```python
from build123d import *
from build123d.topology import SkipClean

# Parameters (mm, degrees)
SKETCH1_R               = 3.429
SKETCH1_R_2             = 2.286
BOSS_EXTRUDE1_DEPTH     = 3.556
BOSS_EXTRUDE2_START     = -1.27
BOSS_EXTRUDE2_DEPTH     = 1.27
BOSS_EXTRUDE3_START     = -1.27
SKETCH2_3_R             = 2.286
SKETCH2_3_R_2           = 1.27
BOSS_EXTRUDE3_DEPTH     = 0.254
SKETCH3_R               = 0.508
CUT_EXTRUDE1_DEPTH      = 17.020635974
LPATTERN1_COUNT         = 6
LPATTERN1_PITCH         = 1.778
CUT_EXTRUDE2_DEPTH      = 17.020635974
CUT_EXTRUDE2_DEPTH_BACK = 17.020635974
SKETCH4_W               = 4.326879353
SKETCH4_H               = 6.724216597
BOSS_EXTRUDE4_START     = 2.286
SKETCH5_R               = 0.508
BOSS_EXTRUDE4_DEPTH     = 1.27
COMBINE1_OUTLINE_R      = 0.508
COMBINE1_OUTLINE_R_2    = 1.27
COMBINE1_DEPTH          = 3.556
SKETCH6_W               = 6.35
SKETCH6_H               = 12.7
BOSS_EXTRUDE5_DEPTH     = 1.27
BOSS_EXTRUDE6_START     = -1.27
SKETCH6_2_W             = 6.35
SKETCH6_2_H             = 12.7
BOSS_EXTRUDE6_DEPTH     = 1.27
FILLET1_R               = 1.27


# Read off the part's stored shape, not the designer's step: Combine1
with BuildPart() as part:
    # Sketch1 → Boss-Extrude1 (new body)
    with BuildSketch(Plane(origin=(0, 0, 0), x_dir=(1, 0, 0), z_dir=(0, 1, 0))):
        with Locations(Location((0, 0, 0), (0, 0, 270))):
            Circle(SKETCH1_R)
        with Locations(Location((0, 0, 0), (0, 0, 270))):
            Circle(SKETCH1_R_2, mode=Mode.SUBTRACT)
    extrude(amount=BOSS_EXTRUDE1_DEPTH)

    # Sketch2 → Boss-Extrude2 (add)
    with BuildSketch(Plane(origin=(0, 3.556, 0), x_dir=(1, 0, 0), z_dir=(0, 1, 0)).offset(BOSS_EXTRUDE2_START)):
        with BuildLine():
            ThreePointArc((-2.54, 2.303571358), (-1.389081498, 3.135042837), (0, 3.429))
            Line((0, 3.429), (0, 15.24))
            ThreePointArc((0, 15.24), (-0.835660201, 14.92028345), (-1.244511661, 14.124427226))
            Line((-1.244511661, 14.124427226), (-2.54, 2.303571358))
        make_face()
        with BuildLine():
            Line((0, 15.24), (0, 3.429))
            ThreePointArc((0, 3.429), (1.389081498, 3.135042837), (2.54, 2.303571358))
            Line((2.54, 2.303571358), (1.244511661, 14.124427226))
            ThreePointArc((1.244511661, 14.124427226), (0.835660201, 14.92028345), (0, 15.24))
        make_face()
    extrude(amount=BOSS_EXTRUDE2_DEPTH)

    # Sketch2<3> → Boss-Extrude3 (add)
    with BuildSketch(Plane(origin=(0, 3.556, 0), x_dir=(1, 0, 0), z_dir=(0, 1, 0)).offset(BOSS_EXTRUDE3_START)):
        with Locations(Location((0, 0, 0), (0, 0, 270))):
            Circle(SKETCH2_3_R)
        with Locations(Location((0, 0, 0), (0, 0, 270))):
            Circle(SKETCH2_3_R_2, mode=Mode.SUBTRACT)
    extrude(amount=BOSS_EXTRUDE3_DEPTH)

    # Sketch3 → Cut-Extrude1 (cut, through all)
    with BuildSketch(Plane(origin=(0, 3.556, 0), x_dir=(1, 0, 0), z_dir=(0, 1, 0))):
        with Locations(Location((0, 5.08, 0), (0, 0, 270))):
            Circle(SKETCH3_R)
    cut_extrude1 = extrude(amount=-CUT_EXTRUDE1_DEPTH, mode=Mode.SUBTRACT)

    # LPattern1: Cut-Extrude1 ×6
    with Locations(*[(0, 0, -i * LPATTERN1_PITCH) for i in range(1, LPATTERN1_COUNT)]):
        add(cut_extrude1, mode=Mode.SUBTRACT)

    # Sketch4 → Cut-Extrude2 (cut, two sides: drawn at the far end of the back side and taken through both)
    with BuildSketch(Plane(origin=(0, 0, 0), x_dir=(0, 0, -1), z_dir=(1, 0, 0)).offset(-CUT_EXTRUDE2_DEPTH_BACK)):
        with Locations((-2.163439677, 3.362108299)):
            Rectangle(SKETCH4_W, SKETCH4_H)
    extrude(amount=CUT_EXTRUDE2_DEPTH + CUT_EXTRUDE2_DEPTH_BACK, mode=Mode.SUBTRACT)

    # Mirror1: part across plane


with BuildPart() as part_1:
    with SkipClean():  # the faces are left unmerged after this step: merging them gives an invalid solid
        add(part.part)
        add(part.part.mirror(Plane.XY))


with BuildPart() as body_2:
    # Sketch5 → Boss-Extrude4 (new body)
    with BuildSketch(Plane(origin=(0, 0, 0), x_dir=(1, 0, 0), z_dir=(0, 1, 0)).offset(BOSS_EXTRUDE4_START)):
        Polygon((3.175, 16.51), (15.875, 12.7), (3.175, 8.89), (3.175, 3.81), (-3.175, 3.81), (-3.175, 16.51), align=None)
        with Locations(Location((4.191, 12.7, 0), (0, 0, 270))):
            Circle(SKETCH5_R, mode=Mode.SUBTRACT)
        with Locations(Location((5.969, 12.7, 0), (0, 0, 270))):
            Circle(SKETCH5_R, mode=Mode.SUBTRACT)
        with Locations(Location((7.747, 12.7, 0), (0, 0, 270))):
            Circle(SKETCH5_R, mode=Mode.SUBTRACT)
        with Locations(Location((9.525, 12.7, 0), (0, 0, 270))):
            Circle(SKETCH5_R, mode=Mode.SUBTRACT)
        with Locations(Location((11.303, 12.7, 0), (0, 0, 270))):
            Circle(SKETCH5_R, mode=Mode.SUBTRACT)
    extrude(amount=BOSS_EXTRUDE4_DEPTH)


with BuildPart() as combine1_tool:
    # Combine1 outline → Combine1 (new body)
    with BuildSketch(Plane(origin=(0, 0, 0), x_dir=(1, 0, 0), z_dir=(0, 1, 0))):
        with BuildLine():
            ThreePointArc((2.54, -2.303571358), (3.429, 0), (2.54, 2.303571358))
            Line((2.54, 2.303571358), (1.244511661, 14.124427226))
            ThreePointArc((1.244511661, 14.124427226), (0, 15.24), (-1.244511661, 14.124427226))
            Line((-1.244511661, 14.124427226), (-2.54, 2.303571358))
            ThreePointArc((-2.54, 2.303571358), (-3.429, 0), (-2.54, -2.303571358))
            Line((-2.54, -2.303571358), (-1.244511661, -14.124427226))
            ThreePointArc((-1.244511661, -14.124427226), (0, -15.24), (1.244511661, -14.124427226))
            Line((1.244511661, -14.124427226), (2.54, -2.303571358))
        make_face()
        with Locations((0, -5.08)):
            Circle(COMBINE1_OUTLINE_R, mode=Mode.SUBTRACT)
        with Locations((0, -13.97)):
            Circle(COMBINE1_OUTLINE_R, mode=Mode.SUBTRACT)
        with Locations((0, -12.192)):
            Circle(COMBINE1_OUTLINE_R, mode=Mode.SUBTRACT)
        with Locations((0, -10.414)):
            Circle(COMBINE1_OUTLINE_R, mode=Mode.SUBTRACT)
        with Locations((0, -8.636)):
            Circle(COMBINE1_OUTLINE_R, mode=Mode.SUBTRACT)
        with Locations((0, -6.858)):
            Circle(COMBINE1_OUTLINE_R, mode=Mode.SUBTRACT)
        Circle(COMBINE1_OUTLINE_R_2, mode=Mode.SUBTRACT)
    extrude(amount=COMBINE1_DEPTH)


with BuildPart() as part_2:
    add(part_1.part)

    # Combine1: cut by combine1_tool
    add(combine1_tool.part, mode=Mode.SUBTRACT)


with BuildPart() as body_2_1:
    add(body_2.part)

    # Combine1: cut by combine1_tool
    add(combine1_tool.part, mode=Mode.SUBTRACT)

    # Sketch6 → Boss-Extrude5 (add)
    with BuildSketch(Plane.XZ.offset(-2.286)):
        with Locations((0, -10.16)):
            Rectangle(SKETCH6_W, SKETCH6_H)
    extrude(amount=BOSS_EXTRUDE5_DEPTH)

    # Sketch6<2> → Boss-Extrude6 (add)
    with BuildSketch(Plane.XZ.offset(-2.286).offset(BOSS_EXTRUDE6_START)):
        with Locations((0, -10.16)):
            Rectangle(SKETCH6_2_W, SKETCH6_2_H)
    extrude(amount=-BOSS_EXTRUDE6_DEPTH)

    # Fillet1
    fillet1_edges = [body_2_1.edges().sort_by_distance(p)[0] for p in [
        (15.875, 2.921, -12.7),
    ]]
    fillet(fillet1_edges, radius=FILLET1_R)


solid = body_2_1.part
```
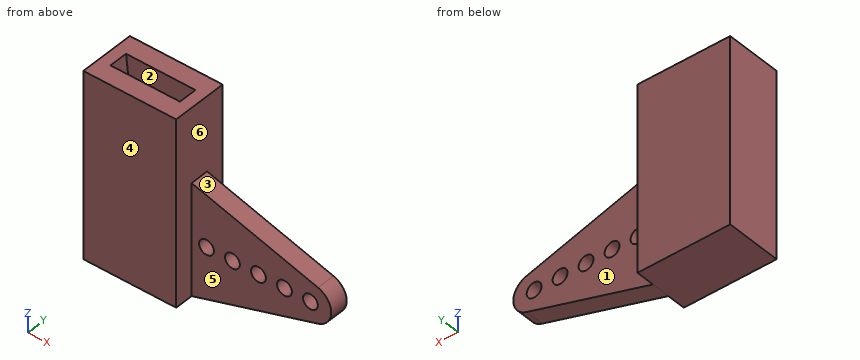
Geometry check sheet. Reference: the model listing, model coordinates, mm. Face numbers are marked on the shaded views. A direction names the side the tool comes from. Coordinates: 2 decimals unless noted, no trailing zeros. Loops run counter-clockwise (first coordinate to the right, second up) from the corner with the lowest first, then second, coordinate; pieces in that order, holes last.
Item 1: Sectioned sample at B-B, the plane y = 3. Record the boundary of the cut face in (x, z) (3 decimals), then the cut area to 3 significant figures.
Item 2: Sectioned sample at C-C, the plane x = 11. Record the boundary of the cut face in (y, z).
Item 3: Go/stop test with flat-tipped pins: pin 1 Ø6 at (x, z) = (9.5, -11.5) entering from +Y; pin 2 Ø1 at (x, y) = (5.5, 3) entering from -Z; pin 3 Ø1.3 at (x, z) = (11.303, -12.7) entering from -Y. Record where each tip stops, or that it passes through.
Item 4: Access from +Z, -Z, +X, -X, +Y, -Y to the whole of each face (thin tool, end or side, straight path). Record for the marked faces 4, 5 and 6.
Item 5: Thickness scan on line 1 (Y direction, x = 0.75, z = -6.75); line 2 (Y direction, x = 3.75, z = -10.75); line 3 (X direction, y = 1.8, z = -15.5) (3 decimals). Record the ranges inside material, lowest first.
Item 6: Sectioned sample at D-D, the plane z = -6.5. Record the boundary of the cut face in (x, y) (3 decimals), then the cut area to 3 significant figures.
Item 7: Release check for a two-part mould opening along X. For the marked faces 1, 2 and 3 record: released by +X, released by -X, zero draft, split by the parting line, or undercut.
Item 8: Sectioned sample at A-A, the plane z = -12.7. Count the separate pieces of the cut face and the enclosed holes in it, then the cut area to 3 significant figures.
Check result:
1. outline: (-3.175, -16.51) - (3.175, -16.51) - (11.82, -13.916) arc R1.27 ccw to (11.82, -11.484) - (3.175, -8.89) - (3.175, -3.81) - (2.375, -3.81) - (1.245, -14.124) arc R1.252 cw to (-1.245, -14.124) - (-2.375, -3.81) - (-3.175, -3.81) - close; hole circle Ø1.016 at (4.191, -12.7); hole circle Ø1.016 at (5.969, -12.7); hole circle Ø1.016 at (7.747, -12.7); hole circle Ø1.016 at (9.525, -12.7); hole circle Ø1.016 at (11.303, -12.7)
1. area: 82.2 mm2
2. outline: (2.29, -14.16) - (3.56, -14.16) - (3.56, -13.11) - (2.29, -13.11) - close; (2.29, -12.29) - (3.56, -12.29) - (3.56, -11.24) - (2.29, -11.24) - close
3. pin 1: stops at y = 3.56
3. pin 2: stops at z = -15.96
3. pin 3: stops at y = 2.29
4. face 4: +Z, -Z, +X, -X, -Y
4. face 5: +Z, -Z, +X, -Y
4. face 6: +Z, +X
5. line 1: y = 1.02 to 2.29, 3.56 to 4.83
5. line 2: y = 2.29 to 3.56
5. line 3: x = -3.175 to 3.175
6. outline: (-3.175, 1.016) - (3.175, 1.016) - (3.175, 4.826) - (-3.175, 4.826) - close; hole (-2.08, 2.286) - (2.08, 2.286) - (2.08, 3.556) - (-2.08, 3.556) - close
6. area: 18.9 mm2
7. face 1: zero draft
7. face 2: undercut
7. face 3: released by +X
8. separate pieces: 6
8. enclosed holes: 1
8. area: 26.3 mm2
